Input: part model. Units: mm. Frame: model coordinates. A direction names the side the tool comes from. Give positions to 0.01 mm unless a question says otherwise; leave off trailing zeros. Order: outer loops, then holes, each group sorted by start corner. A loop starts at its lowest first (then second) coordinate and runs counter-clockwise, first axis right, second up.
```python
from build123d import *

# Parameters (mm, degrees)
SKETCH1_W           = 31
SKETCH1_H           = 42.5
BOSS_EXTRUDE1_DEPTH = 3
SKETCH2_W           = 37
SKETCH2_H           = 48.5
SKETCH2_W_2         = 31
SKETCH2_H_2         = 42.5
BOSS_EXTRUDE2_DEPTH = 15.6
CUT_EXTRUDE1_REACH  = 36.259
SKETCH3_R           = 1.65
CUT_EXTRUDE2_REACH  = 56.202
SKETCH4_W           = 21.4
SKETCH4_H           = 12.6
CUT_EXTRUDE3_REACH  = 56.202
SKETCH5_W           = 10
SKETCH5_H           = 10.6
CUT_EXTRUDE5_REACH  = 36.259
FILLET4_R           = 1
FILLET1_R           = 3


with BuildPart() as part:
    # Sketch1 → Boss-Extrude1 (new body)
    with BuildSketch(Plane.XY):
        Rectangle(SKETCH1_W, SKETCH1_H)
    extrude(amount=BOSS_EXTRUDE1_DEPTH)

    # Sketch2 → Boss-Extrude2 (add)
    with BuildSketch(Plane.XY):
        Rectangle(SKETCH2_W, SKETCH2_H)
        Rectangle(SKETCH2_W_2, SKETCH2_H_2, mode=Mode.SUBTRACT)
    extrude(amount=BOSS_EXTRUDE2_DEPTH)

    # Sketch3 → Cut-Extrude1 (cut, up to next)
    with BuildSketch(Plane(origin=(0, 0, 0), x_dir=(-1, 0, 0), z_dir=(0, 0, -1)), mode=Mode.PRIVATE) as cut_extrude1_sk1:
        with Locations((12.35, 18.6)):
            Circle(SKETCH3_R)
    cut_extrude1_tool1 = extrude(cut_extrude1_sk1.sketch, amount=-CUT_EXTRUDE1_REACH, mode=Mode.PRIVATE) & part.part
    # Sketch3 → Cut-Extrude1 (cut, up to next)
    with BuildSketch(Plane(origin=(0, 0, 0), x_dir=(-1, 0, 0), z_dir=(0, 0, -1)), mode=Mode.PRIVATE) as cut_extrude1_sk2:
        with Locations((0, -18.6)):
            Circle(SKETCH3_R)
    cut_extrude1_tool2 = extrude(cut_extrude1_sk2.sketch, amount=-CUT_EXTRUDE1_REACH, mode=Mode.PRIVATE) & part.part
    cut_extrude1_1 = cut_extrude1_tool1.solids().sort_by_distance((-12.35, 18.6, 0))[0]
    add(cut_extrude1_1, mode=Mode.SUBTRACT)
    cut_extrude1_2 = cut_extrude1_tool2.solids().sort_by_distance((0, -18.6, 0))[0]
    add(cut_extrude1_2, mode=Mode.SUBTRACT)
    cut_extrude1 = cut_extrude1_1 + cut_extrude1_2  # Cut-Extrude1 as one shape, for the pattern or mirror that repeats it

    # Mirror1: Cut-Extrude1 across plane
    add(cut_extrude1.mirror(Plane(origin=(0, 0, 0), x_dir=(0, 0, 1), z_dir=(1, 0, 0))), mode=Mode.SUBTRACT)

    # Sketch4 → Cut-Extrude2 (cut, up to next)
    with BuildSketch(Plane(origin=(0, 24.25, 0), x_dir=(1, 0, 0), z_dir=(0, 1, 0)), mode=Mode.PRIVATE) as cut_extrude2_sk1:
        with Locations((0, -9.3)):
            Rectangle(SKETCH4_W, SKETCH4_H)
    cut_extrude2_tool1 = extrude(cut_extrude2_sk1.sketch, amount=-CUT_EXTRUDE2_REACH, mode=Mode.PRIVATE) & part.part
    add(cut_extrude2_tool1.solids().sort_by_distance((0, 24.25, 9.3))[0], mode=Mode.SUBTRACT)

    # Sketch5 → Cut-Extrude3 (cut, up to next)
    with BuildSketch(Plane.XZ.offset(24.25), mode=Mode.PRIVATE) as cut_extrude3_sk1:
        with Locations((10.5, 10.3)):
            Rectangle(SKETCH5_W, SKETCH5_H)
    cut_extrude3_tool1 = extrude(cut_extrude3_sk1.sketch, amount=-CUT_EXTRUDE3_REACH, mode=Mode.PRIVATE) & part.part
    cut_extrude3 = cut_extrude3_tool1.solids().sort_by_distance((10.5, -24.25, 10.3))[0]
    add(cut_extrude3, mode=Mode.SUBTRACT)

    # Mirror2: Cut-Extrude3 across plane
    add(cut_extrude3.mirror(Plane(origin=(0, 0, 0), x_dir=(0, 0, 1), z_dir=(1, 0, 0))), mode=Mode.SUBTRACT)

    # Cut-Extrude5: up to this face of the body (flat: up to its plane)
    cut_extrude5_end = Plane(part.part.faces().sort_by_distance((0, 0.959753002, 3))[0])
    # Sketch6 → Cut-Extrude5 (cut, up to the picked face)
    with BuildSketch(Plane.XY.offset(15.6), mode=Mode.PRIVATE) as cut_extrude5_sk1:
        with BuildLine():
            Line((5.5, -21.25), (-5.5, -21.25))
            ThreePointArc((-5.5, -21.25), (0, -22.021115477), (5.5, -21.25))
        make_face()
    cut_extrude5_tool1 = split(extrude(cut_extrude5_sk1.sketch, amount=-CUT_EXTRUDE5_REACH, mode=Mode.PRIVATE), bisect_by=cut_extrude5_end, keep=Keep.BOTH, mode=Mode.PRIVATE)
    add(cut_extrude5_tool1.solids().sort_by(Axis((0, -21.558962, 15.6), (0, 0, -1)))[0], mode=Mode.SUBTRACT)

    # Fillet4
    fillet4_edges = [part.edges().sort_by_distance(p)[0] for p in [
        (0, -24.25, 0),
        (-18.5, -24.25, 7.8),
        (18.5, 0, 0),
        (18.5, -24.25, 7.8),
        (0, 24.25, 0),
        (18.5, 24.25, 7.8),
        (-18.5, 0, 0),
        (-18.5, 24.25, 7.8),
    ]]
    fillet(fillet4_edges, radius=FILLET4_R)

    # Fillet1
    fillet1_edges = [part.edges().sort_by_distance(p)[0] for p in [
        (10.7, 22.75, 3),
        (-10.7, 22.75, 3),
        (15.5, -22.75, 5),
        (5.5, -22.75, 5),
        (-5.5, -22.75, 5),
        (-15.5, -22.75, 5),
    ]]
    fillet(fillet1_edges, radius=FILLET1_R)


solid = part.part
```
1) Pull-direction query (Y, two-part tool) for faces 1 (the face through (0.4, -20.2, 1.5)), 2 (the face through (10, -21.25, 4)), 3 (the face through (18.199, -23.965, 8.402)), 4 (the face through (9.84, 22.73, 3.9)); classes: pulls with the +Y half, pulls with the -Y half, needs draft (parallel to the pull), parting line crosses it, or undercut.
2) Reachability of faces 5 (the face through (-13, 21.25, 9)), 6 (the face through (10.7, 23, 11)), 7 (the face through (14.64, -22.73, 5.9)) from +Z, -Z, +X, -X, +Y, -Y: full face, straight path, thin tool, end or side. Return the list, or none.
3) Cut plane A-A (y = 18.6). Return the cut outline in (x, z), then the cut area to 3 significant figures.
4) First-contact query: P1, Ø3, axis at x = 5, z = 8, coming from the +Y side; P2, Ø2.5, axis at x = -12.35, y = 18.6, coming from the +Z side; P3, Ø0.9, axis at x = 10, y = -23, coming from the +Z side; P4, Ø2.5, axis at x = -12, z = 7, coming from the -Y side. Flat tips, straight axial feed; report the tip coordinate or a pass-through.
5) Cut plane D-D (y = -4). Return the cut outline in (x, z).
6) Cut plane B-B (x = 0.5). Return the cut outline in (y, z).
7) Line query: probe 1 along X at (y, z) = (-11, 10.5); probe 2 along X at (y, z) = (-18.6, 1.3); probe 3 along Y at (x, z) = (-12, 3.5). Output: solid intervals per line, ascending.
8) Cut plane C-C (y = -18.6). Return the cut outline in (x, z), then the cut area to 3 significant figures.
Geometry says:
1. face 1: undercut
1. face 2: undercut
1. face 3: pulls with the -Y half
1. face 4: needs draft
2. face 5: +Z
2. face 6: +Z, +Y, -Y
2. face 7: +Z, -Y
3. outline: (-18.5, 1) arc R1 ccw to (-17.5, 0) - (-14, 0) - (-14, 3) - (-15.5, 3) - (-15.5, 15.6) - (-18.5, 15.6) - close; (-10.7, 0) - (10.7, 0) - (10.7, 3) - (-10.7, 3) - close; (14, 0) - (17.5, 0) arc R1 ccw to (18.5, 1) - (18.5, 15.6) - (15.5, 15.6) - (15.5, 3) - (14, 3) - close
3. area: 166 mm2
4. P1: stops at y = -21.25
4. P2: passes through
4. P3: stops at z = 5
4. P4: stops at y = 21.25
5. outline: (-18.5, 1) arc R1 ccw to (-17.5, 0) - (17.5, 0) arc R1 ccw to (18.5, 1) - (18.5, 15.6) - (15.5, 15.6) - (15.5, 3) - (-15.5, 3) - (-15.5, 15.6) - (-18.5, 15.6) - close
6. outline: (-24.25, 1) arc R1 ccw to (-23.25, 0) - (-20.17, 0) - (-20.17, 3) - (-22.01, 3) - (-22.01, 15.6) - (-24.25, 15.6) - close; (-17.03, 0) - (23.25, 0) arc R1 ccw to (24.25, 1) - (24.25, 3) - (-17.03, 3) - close
7. probe 1: x = -18.5 to -15.5, 15.5 to 18.5
7. probe 2: x = -18.5 to -1.65, 1.65 to 18.5
7. probe 3: y = -24.25 to -21.25, 21.25 to 24.25
8. outline: (-18.5, 1) arc R1 ccw to (-17.5, 0) - (-1.65, 0) - (-1.65, 3) - (-15.5, 3) - (-15.5, 15.6) - (-18.5, 15.6) - close; (1.65, 0) - (17.5, 0) arc R1 ccw to (18.5, 1) - (18.5, 15.6) - (15.5, 15.6) - (15.5, 3) - (1.65, 3) - close
8. area: 176 mm2
